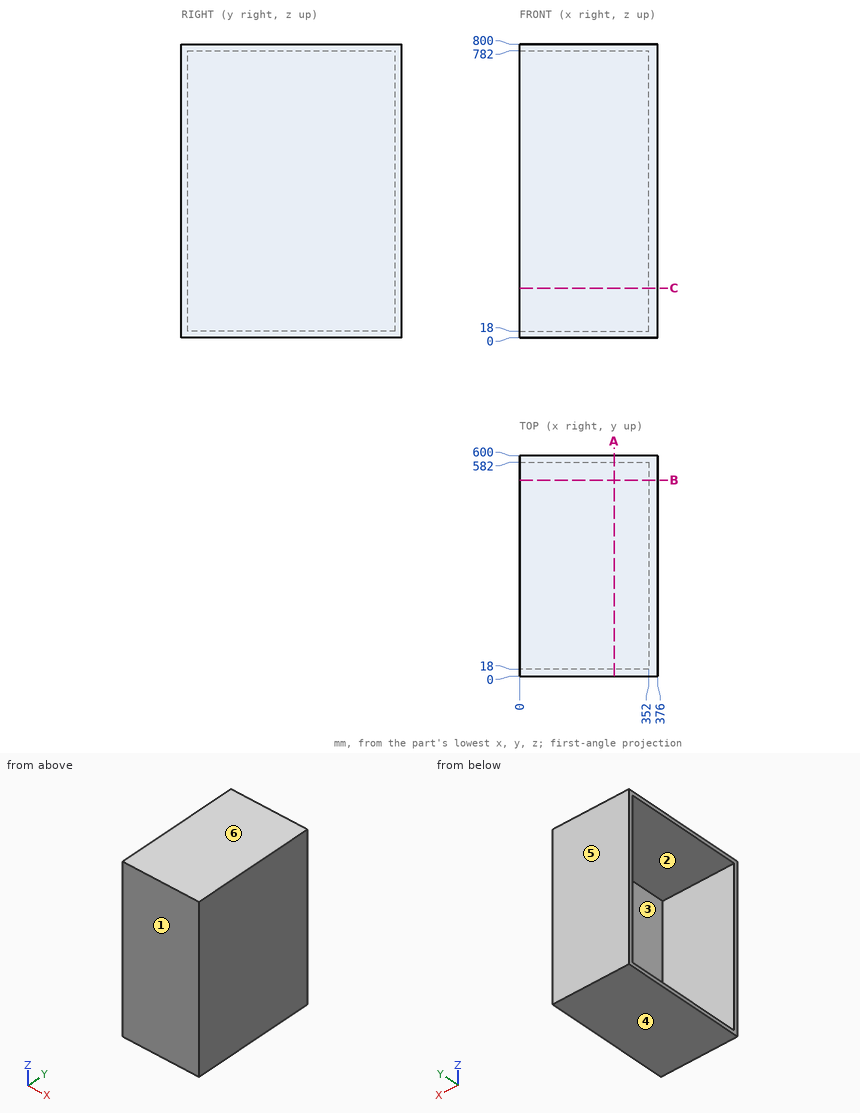
Check sheet for the drawn part. Datum: minimum x, y, z corner. Units: mm. A direction names the side the tool comes from. Give positions to 0.01 mm unless a question says otherwise; leave off trailing zeros. Write each loop counter-clockwise with the first axis right and the second up, starting at its lowest first coordinate (ties: lowest second). Pieces come first, ordered by that corner, then holes. Notation, with made-up numbers: M 2.25,14 L 19.25,14 A22 cw 19.25,23 Z; hole C -10.75,60.5 d11. An arc over 180 degrees is marked long. One line per question, with ' | ' between items.
1) Thickness scan on line 1 along Y through (x, z) = (181, 641.5); line 2 along Z through (x, y) = (167.5, 508); line 3 along X through (y, z) = (82, 264). Record the ranges inside material, lowest first. Write a range as [from, to].
Result:
line 1: y = [0, 18], [582, 600] | line 2: z = [0, 18], [782, 800] | line 3: x = [352, 376]
2) Section check C-C on z = 135. Enter the section's corners in (x, y), plus the area to 3 significant figures.
Result:
outline: M 0,0 L 376,0 L 376,600 L 0,600 L 0,582 L 352,582 L 352,18 L 0,18 Z | area: 27,100 mm2
3) Section check A-A on x = 257.5. Enter the section's corners in (y, z).
Result:
outline: M 0,0 L 600,0 L 600,800 L 0,800 Z; hole M 18,18 L 582,18 L 582,782 L 18,782 Z
4) Gauge pin test, flat end, axial feed: pin 1 Ø5 at (y, z) = (522, 375) entering from -X. Record the tip position at first contact, or that the pin passes through.
Result:
pin 1: stops at x = 352
5) Section check B-B on y = 533.5. Enter the section's corners in (x, z).
Result:
outline: M 0,0 L 376,0 L 376,800 L 0,800 L 0,782 L 352,782 L 352,18 L 0,18 Z
6) Mould release check, pull along Z, two halves, no side actions. Record for the marked faces 3, 4, 5 and 6: released by +Z, released by -Z, zero draft, split by the parting line, or undercut.
Result:
face 3: undercut | face 4: released by -Z | face 5: zero draft | face 6: released by +Z
7) Set-up check for the marked faces 1 and 2: record each of +Z, -Z, +X, -X, +Y, -Y from which the full face is reachable in a straight line by a thin tool's end or side.
Result:
face 1: +Z, -Z, +X, -X, -Y | face 2: -X
